Design review of the part built by this model. Coordinates are the model's own, in mm. Coordinates: 2 decimals unless noted, no trailing zeros. Write each loop counter-clockwise with the first axis right and the second up, starting at its lowest first coordinate (ties: lowest second). Pieces come first, ordered by that corner, then holes. Notation, with made-up numbers: (37, 73.5) - (50, 73.5) arc R5 ccw to (50, 80.5) - close; hole circle Ø9 at (2.25, -17). An arc over 180 degrees is marked (long way). One line per item, written item: value.
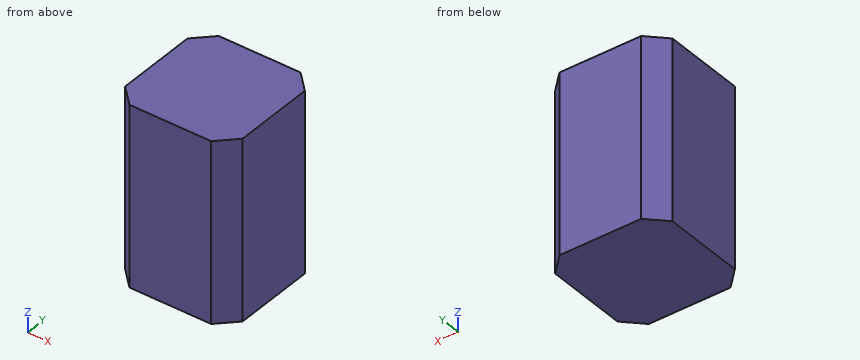
from build123d import *

# Parameters (mm, degrees)
EXTRUDE_2_DEPTH = 237
SCALE_1_SCALE   = 0.761290323


with BuildPart() as part:
    # 草图3 → 凸台-拉伸2 (new body)
    with BuildSketch(Plane.XY):
        Polygon((-77.5, -54.021861301), (-54.021861301, -77.5), (54.021861301, -77.5), (77.5, -54.021861301), (77.5, 54.021861301), (54.021861301, 77.5), (-54.021861301, 77.5), (-77.5, 54.021861301), align=None)
    extrude(amount=EXTRUDE_2_DEPTH)


with BuildPart() as part_1:
    # 缩放比例1: scaled about (0, 0, 0)
    add(part.part.scale(SCALE_1_SCALE))


solid = part_1.part
1. Wall thickness on line 1 along Y through (x, z) = (-52, 154.5); line 2 along X through (y, z) = (-47, 77); line 3 along Y through (x, z) = (46, 85): over which ranges is each line inside the solid? List them lowest first.
Answer block:
line 1: y = -48.13 to 48.13
line 2: x = -53.13 to 53.13
line 3: y = -54.13 to 54.13
2. Consider section C-C, the plane x = -48. Write out the cut boundary in (y, z).
Answer block:
outline: (-52.13, 0) - (52.13, 0) - (52.13, 180.43) - (-52.13, 180.43) - close
3. Consider section B-B, the plane y = 45. Write out the cut boundary in (x, z), then the cut area to 3 significant figures.
Answer block:
outline: (-55.13, 0) - (55.13, 0) - (55.13, 180.43) - (-55.13, 180.43) - close
area: 19,900 mm^2
4. Consider section A-A, the plane z = 144.5. Write out the cut boundary in (x, y).
Answer block:
outline: (-59, -41.13) - (-41.13, -59) - (41.13, -59) - (59, -41.13) - (59, 41.13) - (41.13, 59) - (-41.13, 59) - (-59, 41.13) - close
